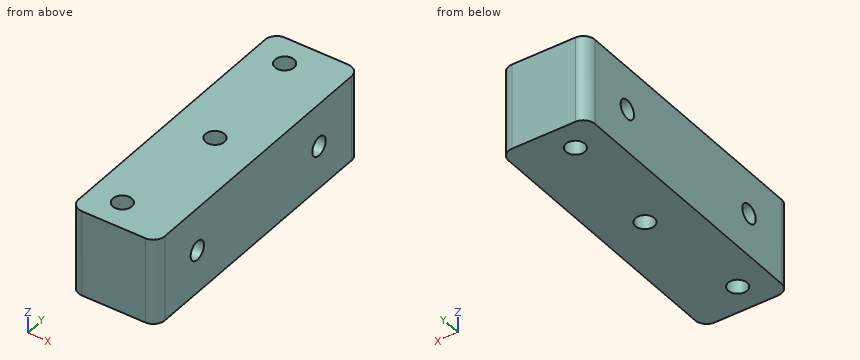
from build123d import *

# Parameters (mm, degrees)
SKETCH_1_W          = 15
SKETCH_1_H          = 50
SKETCH_1_R          = 1.65
EXTRUDE_1_DEPTH     = 15
SKETCH_2_R          = 1.65
CUT_EXTRUDE_1_DEPTH = 15
FILLET_1_R          = 2


with BuildPart() as part:
    # ｽｹｯﾁ1 → ﾎﾞｽ - 押し出し1 (new body)
    with BuildSketch(Plane.XY):
        with Locations((7.5, 25)):
            Rectangle(SKETCH_1_W, SKETCH_1_H)
        with Locations((5.5, 5)):
            Circle(SKETCH_1_R, mode=Mode.SUBTRACT)
        with Locations(Location((5.5, 45, 0), (0, 0, 180))):
            Circle(SKETCH_1_R, mode=Mode.SUBTRACT)
        with Locations((7.5, 25)):
            Circle(SKETCH_1_R, mode=Mode.SUBTRACT)
    extrude(amount=EXTRUDE_1_DEPTH)

    # ｽｹｯﾁ2 → ｶｯﾄ - 押し出し1 (cut)
    with BuildSketch(Plane.ZY):
        with Locations((7.5, 40)):
            Circle(SKETCH_2_R)
        with Locations((7.5, 10)):
            Circle(SKETCH_2_R)
    extrude(amount=-CUT_EXTRUDE_1_DEPTH, mode=Mode.SUBTRACT)

    # ﾌｨﾚｯﾄ1
    fillet_1_edges = [part.edges().sort_by_distance(p)[0] for p in [
        (0, 50, 7.5),
        (15, 50, 7.5),
        (15, 0, 7.5),
        (0, 0, 7.5),
    ]]
    fillet(fillet_1_edges, radius=FILLET_1_R)


solid = part.part
CAD build for the part. Positions are in the model's coordinates, mm. Coordinates: 2 decimals unless noted, no trailing zeros. Order: outer loops, then holes, each group sorted by start corner. A loop starts at its lowest first (then second) coordinate and runs counter-clockwise, first axis right, second up.
Item 1: Band-saw the part on D-D on z = 12. List the corners of the cut face in (x, y).
Check sheet entries:
outline: (0, 2) arc R2 ccw to (2, 0) - (13, 0) arc R2 ccw to (15, 2) - (15, 48) arc R2 ccw to (13, 50) - (2, 50) arc R2 ccw to (0, 48) - close; hole circle Ø3.3 at (5.5, 5); hole circle Ø3.3 at (5.5, 45); hole circle Ø3.3 at (7.5, 25)
Item 2: Band-saw the part on C-C on x = 4.75. List the corners of the cut face in (y, z).
Check sheet entries:
outline: (0, 0) - (3.53, 0) - (3.53, 15) - (0, 15) - close; (6.47, 0) - (43.53, 0) - (43.53, 15) - (6.47, 15) - close; (46.47, 0) - (50, 0) - (50, 15) - (46.47, 15) - close; hole circle Ø3.3 at (10, 7.5); hole circle Ø3.3 at (40, 7.5)
Item 3: Band-saw the part on A-A on z = 7.5. List the corners of the cut face in (x, y).
Check sheet entries:
outline: (0, 2) arc R2 ccw to (2, 0) - (13, 0) arc R2 ccw to (15, 2) - (15, 8.35) - (0, 8.35) - close; (0, 11.65) - (15, 11.65) - (15, 38.35) - (0, 38.35) - close; (0, 41.65) - (15, 41.65) - (15, 48) arc R2 ccw to (13, 50) - (2, 50) arc R2 ccw to (0, 48) - close; hole circle Ø3.3 at (5.5, 5); hole circle Ø3.3 at (5.5, 45); hole circle Ø3.3 at (7.5, 25)
Item 4: Drill centre lines: L1, parallel to Y at x = 5.75, z = 13.5; L2, parallel to Y at x = 11.25, z = 8.75; L3, parallel to Y at x = 5.5, z = 6.5. Where is each one in solid material? Low to high.
Check sheet entries:
L1: y = 0 to 3.37, 6.63 to 43.37, 46.63 to 50
L2: y = 0 to 8.92, 11.08 to 38.92, 41.08 to 50
L3: y = 0 to 3.35, 6.65 to 8.69, 11.31 to 38.69, 41.31 to 43.35, 46.65 to 50
Item 5: Band-saw the part on B-B on y = 5. List the corners of the cut face in (x, z).
Check sheet entries:
outline: (0, 0) - (3.85, 0) - (3.85, 15) - (0, 15) - close; (7.15, 0) - (15, 0) - (15, 15) - (7.15, 15) - close
